Geometry: final body of the model. Coordinates: model frame, mm. Round coordinates to 2 decimals unless told otherwise and drop trailing zeros. Loops run counter-clockwise (first coordinate to the right, second up) from the corner with the lowest first, then second, coordinate; pieces in that order, holes last. Notation, with made-up numbers: M -6.75,-8 L 27.25,-8 A28 ccw 27.25,18 Z; hole C -2,30 d5. An arc over 180 degrees is marked long. Answer as a JSON object with one key per item and string values.
```python
from build123d import *

# Parameters (mm, degrees)
SKETCH2_W           = 57.153
SKETCH2_H           = 38.1011
SKETCH2_H_2         = 19.05
SKETCH2_W_2         = 76.202
SKETCH2_W_3         = 76.203
SKETCH2_W_4         = 76.2019
SKETCH2_W_5         = 19.0499
BOSS_EXTRUDE1_DEPTH = 5


with BuildPart() as part:
    # Sketch2 → Boss-Extrude1 (new body)
    with BuildSketch(Plane(origin=(0, 0, 0), x_dir=(1, 0, 0), z_dir=(0, 1, 0))):
        Polygon((382.958, 164.299), (383.35, 164.284), (383.741, 164.237), (384.126, 164.162), (384.503, 164.055), (384.87, 163.919), (385.226, 163.755), (385.572, 163.564), (385.897, 163.344), (386.203, 163.102), (386.493, 162.834), (386.761, 162.547), (387.004, 162.238), (387.223, 161.913), (387.414, 161.569), (387.576, 161.212), (387.713, 160.845), (387.819, 160.467), (387.897, 160.082), (387.943, 159.693), (387.96, 159.299), (387.96, 5.27237), (387.943, 4.881), (387.897, 4.49104), (387.819, 4.10655), (387.713, 3.72759), (387.576, 3.35966), (387.414, 3.00412), (387.223, 2.66099), (387.004, 2.3344), (386.761, 2.02572), (386.493, 1.73771), (386.203, 1.47037), (385.897, 1.22783), (385.572, 1.0101), (385.226, 0.818554), (384.87, 0.654569), (384.503, 0.518142), (384.126, 0.412034), (383.741, 0.334863), (383.35, 0.289388), (382.958, 0.272852), (5.09598, 0.272852), (4.70186, 0.289388), (4.3119, 0.334863), (3.9274, 0.412034), (3.54983, 0.518142), (3.18189, 0.654569), (2.82498, 0.818554), (2.48185, 1.0101), (2.15663, 1.22783), (1.84795, 1.47037), (1.55994, 1.73771), (1.2926, 2.02572), (1.05006, 2.3344), (0.830957, 2.66099), (0.63941, 3.00412), (0.475424, 3.35966), (0.338998, 3.72759), (0.232888, 4.10655), (0.157097, 4.49104), (0.110243, 4.881), (0.0950846, 5.27375), (0.0950846, 159.299), (0.110243, 159.693), (0.157097, 160.082), (0.232888, 160.467), (0.338998, 160.845), (0.475424, 161.212), (0.63941, 161.569), (0.830957, 161.913), (1.05006, 162.238), (1.2926, 162.547), (1.55994, 162.834), (1.84795, 163.102), (2.15663, 163.344), (2.48185, 163.564), (2.82498, 163.755), (3.18189, 163.919), (3.54983, 164.055), (3.9274, 164.162), (4.3119, 164.237), (4.70186, 164.284), (5.09598, 164.299), align=None)
        Polygon((329.756, 58.4743), (329.756, 39.4243), (310.706, 39.4243), (310.706, 20.3729), (367.859, 20.3729), (367.859, 39.4243), (348.809, 39.4243), (348.809, 58.4743), align=None, mode=Mode.SUBTRACT)
        Polygon((20.1952, 115.624), (20.1952, 77.5243), (20.1938, 77.5243), (20.1938, 39.4229), (20.1952, 39.4229), (20.1952, 20.3729), (305.947, 20.3729), (305.947, 115.624), align=None, mode=Mode.SUBTRACT)
        with Locations((339.2825, 96.57345)):
            Rectangle(SKETCH2_W, SKETCH2_H, mode=Mode.SUBTRACT)
        with Locations((339.2825, 134.674)):
            Rectangle(SKETCH2_W, SKETCH2_H_2, mode=Mode.SUBTRACT)
        with Locations((267.846, 134.674)):
            Rectangle(SKETCH2_W_2, SKETCH2_H_2, mode=Mode.SUBTRACT)
        with Locations((182.1205, 134.674)):
            Rectangle(SKETCH2_W_3, SKETCH2_H_2, mode=Mode.SUBTRACT)
        with Locations((96.39605, 134.674)):
            Rectangle(SKETCH2_W_4, SKETCH2_H_2, mode=Mode.SUBTRACT)
        with Locations((29.72015, 134.674)):
            Rectangle(SKETCH2_W_5, SKETCH2_H_2, mode=Mode.SUBTRACT)
    extrude(amount=BOSS_EXTRUDE1_DEPTH)


solid = part.part
```
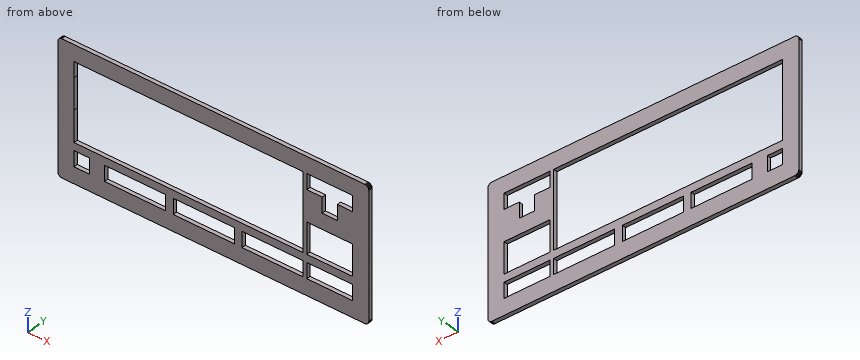
1) Cut plane B-B on x = 45.5. Return the cut outline in (y, z), and give its area (3 significant figures).
Geometry results:
{"outline": "M 0,-164.3 L 5,-164.3 L 5,-115.62 L 0,-115.62 Z; M 0,-20.37 L 5,-20.37 L 5,-0.27 L 0,-0.27 Z", "area": "344 mm2"}
2) Cut plane C-C on x = 250.5. Return the cut outline in (y, z).
Geometry results:
{"outline": "M 0,-164.3 L 5,-164.3 L 5,-144.2 L 0,-144.2 Z; M 0,-125.15 L 5,-125.15 L 5,-115.62 L 0,-115.62 Z; M 0,-20.37 L 5,-20.37 L 5,-0.27 L 0,-0.27 Z"}
3) Cut plane D-D on x = 359. Return the cut outline in (y, z).
Geometry results:
{"outline": "M 0,-164.3 L 5,-164.3 L 5,-144.2 L 0,-144.2 Z; M 0,-125.15 L 5,-125.15 L 5,-115.62 L 0,-115.62 Z; M 0,-77.52 L 5,-77.52 L 5,-39.42 L 0,-39.42 Z; M 0,-20.37 L 5,-20.37 L 5,-0.27 L 0,-0.27 Z"}
4) Cut plane A-A on z = -46.5. Return the cut outline in (x, y).
Geometry results:
{"outline": "M 0.1,0 L 20.19,0 L 20.19,5 L 0.1,5 Z; M 305.95,0 L 329.76,0 L 329.76,5 L 305.95,5 Z; M 348.81,0 L 387.96,0 L 387.96,5 L 348.81,5 Z"}
5) Line query: probe 1 along X at (y, z) = (3.8, -102); probe 2 along X at (y, z) = (1, -131.5) (3 decimals); probe 3 along Z at (x, y) = (93, 2.6). Output: solid intervals per line, ascending.
Geometry results:
{"probe 1": "0.1 to 20.2, 305.95 to 310.71, 367.86 to 387.96", "probe 2": "0.095 to 20.195, 39.245 to 58.295, 134.497 to 144.019, 220.222 to 229.745, 305.947 to 310.706, 367.859 to 387.96", "probe 3": "-164.3 to -144.2, -125.15 to -115.62, -20.37 to -0.27"}
